The drawing under review shows one solid part. Ordinate dimensions are in mm from its lowest x, y, z. A direction names the side the tool comes from. Round coordinates to 2 decimals unless told otherwise and drop trailing zeros. Loops run counter-clockwise (first coordinate to the right, second up) from the corner with the lowest first, then second, coordinate; pieces in that order, holes last. Notation, with made-up numbers: M -17.5,0 L 31.5,0 A18 ccw 31.5,26 Z; hole C 7.5,21.25 d7. An arc over 180 degrees is marked long. Use a Markdown table: item, result.
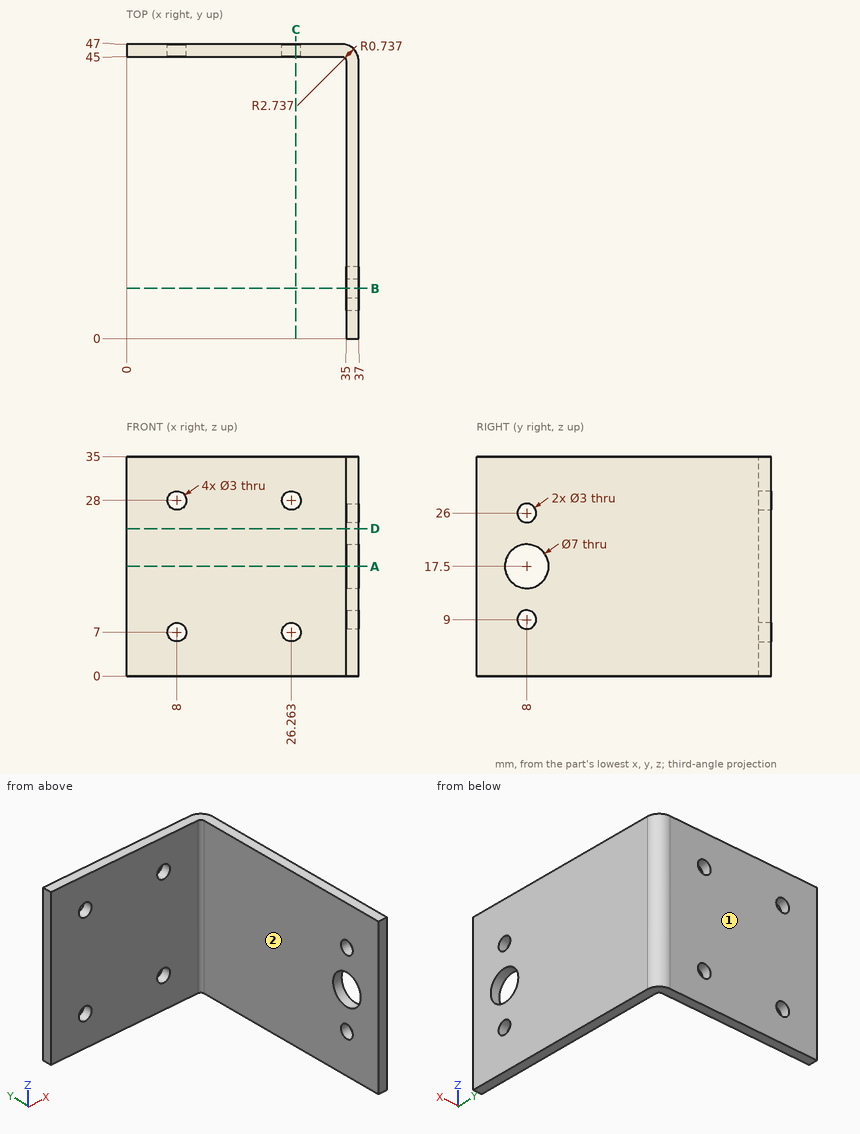
1. Take a section at C-C on x = 27. Give the boundary of the cut face in (y, z).
Check values:
| item | result |
|---|---|
| outline | M 45,0 L 47,0 L 47,5.69 L 45,5.69 Z; M 45,8.31 L 47,8.31 L 47,26.69 L 45,26.69 Z; M 45,29.31 L 47,29.31 L 47,35 L 45,35 Z |
2. Insertion check: pin 1 (2.5 mm diameter, centred on x = 8, z = 7, fed in from -Y); pin 2 (17 mm diameter, centred on x = 18, z = 20, fed in from -Y); pin 3 (5 mm diameter, centred on y = 8, z = 9, fed in from -X). Each pin has a flat end and moves straight along its axis. Give the tip position at first contact, or say it passes through.
Check values:
| item | result |
|---|---|
| pin 1 | passes through |
| pin 2 | stops at y = 45 |
| pin 3 | stops at x = 35 |
3. Take a section at A-A on z = 17.5. Give the boundary of the cut face in (x, y).
Check values:
| item | result |
|---|---|
| outline | M 0,45 L 34.26,45 A0.74 cw 35,44.26 L 35,11.5 L 37,11.5 L 37,44.26 A2.74 ccw 34.26,47 L 0,47 Z; M 35,0 L 37,0 L 37,4.5 L 35,4.5 Z |
4. Take a section at D-D on z = 23.5. Give the boundary of the cut face in (x, y).
Check values:
| item | result |
|---|---|
| outline | M 0,45 L 34.26,45 A0.74 cw 35,44.26 L 35,0 L 37,0 L 37,44.26 A2.74 ccw 34.26,47 L 0,47 Z |
5. Machinability: for the marked faces 1 and 2, which of the approach directions +Z, -Z, +X, -X, +Y, -Y give a long, thin tool a straight path to every point of the face, cutting with its end or side? Answer none if there is none.
Check values:
| item | result |
|---|---|
| face 1 | +Z, -Z, +X, -X, +Y |
| face 2 | +Z, -Z, -X, -Y |
6. Wall thickness on line 1 along Z through (x, y) = (35.75, 8); line 2 along X through (y, z) = (45.85, 28) (1 decimal); line 3 along Y through (x, z) = (23, 33.5): over which ranges is each line inside the solid? List them lowest first. Write a range as from..to.
Check values:
| item | result |
|---|---|
| line 1 | z = 0..7.5, 10.5..14, 21..24.5, 27.5..35 |
| line 2 | x = 0..6.5, 9.5..24.8, 27.8..36.5 |
| line 3 | y = 45..47 |
7. Take a section at B-B on y = 8. Give the boundary of the cut face in (x, z).
Check values:
| item | result |
|---|---|
| outline | M 35,0 L 37,0 L 37,7.5 L 35,7.5 Z; M 35,10.5 L 37,10.5 L 37,14 L 35,14 Z; M 35,21 L 37,21 L 37,24.5 L 35,24.5 Z; M 35,27.5 L 37,27.5 L 37,35 L 35,35 Z |
